Work out the finished part from the listing and answer in its coordinate system (mm). A direction names the side the tool comes from. Round coordinates to 2 decimals unless told otherwise and drop trailing zeros. Write each loop counter-clockwise with the first axis right and the second up, starting at its lowest first coordinate (ties: lowest second). Pieces come first, ordered by that corner, then holes.
1. Find section D-D (z = 17.25). Write down the section's boundary in (x, y).
2. Find section C-C (y = -5.5). Write down the section's boundary in (x, z) (3 decimals), and give its area (3 significant figures).
3. Find section B-B (x = 0). Write down the section's boundary in (y, z) (3 decimals), and give its area (3 significant figures).
4. Flat-ended cylindrical pins translate along their axes: pin 1 Ø3.5 at (x, y) = (20.32, 20.32) entering from -Z; pin 2 Ø3 at (y, z) = (7, 17) entering from +X; pin 3 Ø4 at (x, y) = (-12.5, -18.5) entering from +Z (3 decimals); pin 4 Ø10 at (x, z) = (14, 17.5) entering from -Y. Find the tip coordinate at first contact, or state that the pin passes through.
5. Determine the mould class of faces 1 (the face through (25.4, 0, 2)), 2 (the face through (18.82, 18.95, 1.19)), 3 (the face through (0, 0, 0)), 4 (the face through (-25.4, 0, 2)) for opening direction X: pulls with the +X half, pulls with the -X half, needs draft (parallel to the pull), parting line crosses it, or undercut.
6. Straight lines are drawn through the part: probe 1 along X at (y, z) = (-20.32, 1.7); probe 2 along Z at (x, y) = (0, -11.5). For each, find the intervals that lie inside material, in ascending order.
7. Find section A-A (y = 20.32). Write down the section's boundary in (x, z) (3 decimals).
8. A tool of negligible diameter and unlimited length cuts with its end or side. For faces 5 (the face through (-19.228, 18.607, 1.19)), 6 (the face through (0, -19, 3.175)), 7 (the face through (0, 19, 3.175)), from which of +Z, -Z, +X, -X, +Y, -Y can it reach the whole face along a straight path? Write none if from no direction.
```python
from build123d import *

# Parameters (mm, degrees)
F0_W        = 50.8
F0_H        = 50.8
F1_DEPTH    = 3.175
F3_DEPTH    = 12.7
F4_T1_DEPTH = 29.8470625703
F5_R        = 2.032
F6_DEPTH    = 25.4
F7_SIZE     = 0.762


# Not quite as in the source:
# - a fillet or chamfer that OpenCascade refuses, or shapes differently, is made with other operations: its cross-section is extruded or revolved along the edge and cut away or added


with BuildPart() as f1:
    # F0 (on Top) → F1 (new body)
    with BuildSketch(Plane.XY):
        Rectangle(F0_W, F0_H)
    extrude(amount=F1_DEPTH)

    # F2 (on Front) → F3 (join, symmetric)
    with BuildSketch(Plane.XZ):
        with BuildLine():
            ThreePointArc((8.3472917764, 20.193), (0, 6.477), (-8.3472917764, 20.193))
            Line((-8.3472917764, 20.193), (-25.4, 3.175))
            Line((-25.4, 3.175), (25.4, 3.175))
            Line((25.4, 3.175), (8.3472917764, 20.193))
        make_face()
    extrude(amount=F3_DEPTH, both=True)

    # F4: chamfer of 1.016 on 2 edges, made by hand

    # F4_s2 → F4_t1 (cut)
    with BuildSketch(Plane.XZ.offset(-14.9235312851)):
        with BuildLine():
            Line((-9.00434009, 19.5935484726), (-8.6781133788, 19.3772721718))
            Line((-8.6781133788, 19.3772721718), (-8.659276653, 19.3696511377))
            ThreePointArc((-8.659276653, 19.3696511377), (-8.5217005097, 19.7892691023), (-8.3292435779, 20.1836637838))
            Line((-8.3292435779, 20.1836637838), (-8.3616455415, 20.2073830396))
            ThreePointArc((-8.3616455415, 20.2073830396), (-8.6761048617, 19.893563754), (-9.0186938551, 19.6079315122))
            Line((-9.0186938551, 19.6079315122), (-9.00434009, 19.5935484726))
        make_face()
        with BuildLine():
            Line((9.00434009, 19.5935484726), (8.6781133788, 19.3772721718))
            Line((8.6781133788, 19.3772721718), (8.659276653, 19.3696511377))
            ThreePointArc((8.659276653, 19.3696511377), (8.5217005097, 19.7892691023), (8.3292435779, 20.1836637838))
            Line((8.3292435779, 20.1836637838), (8.3616455415, 20.2073830396))
            ThreePointArc((8.3616455415, 20.2073830396), (8.6761048617, 19.893563754), (9.0186938551, 19.6079315122))
            Line((9.0186938551, 19.6079315122), (9.00434009, 19.5935484726))
        make_face()
    extrude(amount=F4_T1_DEPTH, mode=Mode.SUBTRACT)

    # F5 (on face) → F6 (cut)
    with BuildSketch(Plane(origin=(0, 0, 0), x_dir=(1, 0, 0), z_dir=(0, 0, -1))):
        with Locations((-20.32, 20.32)):
            Circle(F5_R)
        with Locations((-20.32, -20.32)):
            Circle(F5_R)
        with Locations((20.32, 20.32)):
            Circle(F5_R)
        with Locations((20.32, -20.32)):
            Circle(F5_R)
    extrude(amount=-F6_DEPTH, mode=Mode.SUBTRACT)

    # F7
    f7_edges = [f1.edges().sort_by_distance(p)[0] for p in [
        (-22.352, -20.32, 3.175),
        (-22.352, 20.32, 3.175),
        (18.288, 20.32, 3.175),
        (18.288, -20.32, 3.175),
    ]]
    chamfer(f7_edges, length=F7_SIZE)


solid = f1.part
```
Worked answers:
1. outline: (-11.3, -12.7) - (-9.3, -12.7) - (-9.3, 12.7) - (-11.3, 12.7) - close; (9.3, -12.7) - (11.3, -12.7) - (11.3, 12.7) - (9.3, 12.7) - close
2. outline: (-25.4, 0) - (25.4, 0) - (25.4, 3.175) - (8.97, 19.571) - (8.712, 19.4) arc R9.398 cw (long way) to (-8.712, 19.4) - (-8.97, 19.571) - (-25.4, 3.175) - close
2. area: 518 mm2
3. outline: (-25.4, 0) - (25.4, 0) - (25.4, 3.175) - (12.7, 3.175) - (12.7, 6.477) - (-12.7, 6.477) - (-12.7, 3.175) - (-25.4, 3.175) - close
3. area: 245 mm2
4. pin 1: passes through
4. pin 2: stops at x = 13.05
4. pin 3: stops at z = 3.175
4. pin 4: stops at y = -12.7
5. face 1: pulls with the +X half
5. face 2: undercut
5. face 3: needs draft
5. face 4: pulls with the -X half
6. probe 1: x = -25.4 to -22.35, -18.29 to 18.29, 22.35 to 25.4
6. probe 2: z = 0 to 6.48
7. outline: (-25.4, 0) - (-22.352, 0) - (-22.352, 2.413) - (-23.114, 3.175) - (-25.4, 3.175) - close; (-18.288, 0) - (18.288, 0) - (18.288, 2.413) - (17.526, 3.175) - (-17.526, 3.175) - (-18.288, 2.413) - close; (22.352, 0) - (25.4, 0) - (25.4, 3.175) - (23.114, 3.175) - (22.352, 2.413) - close
8. face 5: +Z, -Z
8. face 6: +Z, +X, -X, -Y
8. face 7: +Z, +X, -X, +Y
